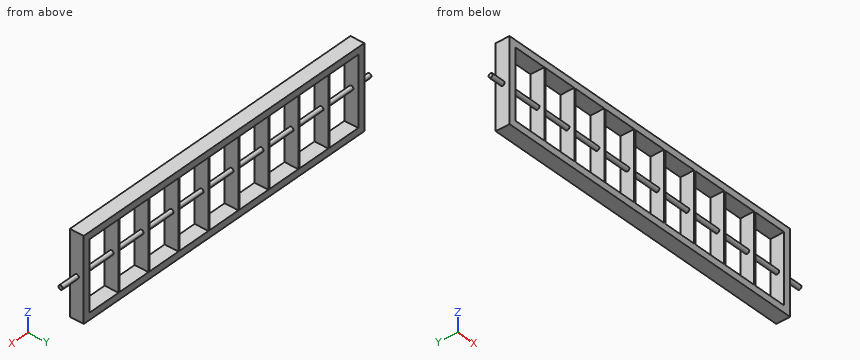
from build123d import *

# Parameters (mm, degrees)
SKETCH1_W                = 468
SKETCH1_H                = 120
SKETCH1_W_2              = 448
SKETCH1_H_2              = 100
BOSS_EXTRUDE1_DEPTH      = 20
SKETCH2_R                = 3
BOSS_EXTRUDE2_DEPTH      = 20
BOSS_EXTRUDE2_DEPTH_BACK = 495
SKETCH4_W                = 2
SKETCH4_H                = 20
BOSS_EXTRUDE3_DEPTH      = 100


with BuildPart() as part:
    # Sketch1 → Boss-Extrude1 (new body)
    with BuildSketch(Plane(origin=(0, 0, 0), x_dir=(1, 0, 0), z_dir=(0, 1, 0))):
        Rectangle(SKETCH1_W, SKETCH1_H)
        Rectangle(SKETCH1_W_2, SKETCH1_H_2, mode=Mode.SUBTRACT)
    extrude(amount=BOSS_EXTRUDE1_DEPTH)

    # Sketch2 → Boss-Extrude2 (add, two sides)
    with BuildSketch(Plane.ZY.offset(234)) as boss_extrude2_sk:
        with Locations((0, 10)):
            Circle(SKETCH2_R)
    extrude(amount=BOSS_EXTRUDE2_DEPTH)
    extrude(boss_extrude2_sk.sketch, amount=-BOSS_EXTRUDE2_DEPTH_BACK)

    # Sketch4 → Boss-Extrude3 (add)
    with BuildSketch(Plane(origin=(0, 0, 50), x_dir=(-1, 0, 0), z_dir=(0, 0, -1))):
        with Locations((-125, 10)):
            Rectangle(SKETCH4_W, SKETCH4_H)
        with Locations((-75, 10)):
            Rectangle(SKETCH4_W, SKETCH4_H)
        with Locations((-25, 10)):
            Rectangle(SKETCH4_W, SKETCH4_H)
        with Locations((25, 10)):
            Rectangle(SKETCH4_W, SKETCH4_H)
        with Locations((75, 10)):
            Rectangle(SKETCH4_W, SKETCH4_H)
        with Locations((125, 10)):
            Rectangle(SKETCH4_W, SKETCH4_H)
        with Locations((175, 10)):
            Rectangle(SKETCH4_W, SKETCH4_H)
        with Locations((-175, 10)):
            Rectangle(SKETCH4_W, SKETCH4_H)
    extrude(amount=BOSS_EXTRUDE3_DEPTH)


solid = part.part
Geometry check sheet. Reference: the model listing, model coordinates, mm. Coordinates: 2 decimals unless noted, no trailing zeros. Write each loop counter-clockwise with the first axis right and the second up, starting at its lowest first coordinate (ties: lowest second). Pieces come first, ordered by that corner, then holes. Notation, with made-up numbers: (-8.75, 74.25) -> (45.25, 74.25) arc R20 cw to (45.25, 82.25) -> close; hole circle Ø5 at (3, 12.5). An arc over 180 degrees is marked (long way). One line per question, with ' | ' between items.
1. Thickness scan on probe 1 along Z at (x, y) = (91, 3); probe 2 along Z at (x, y) = (-188, 12.5); probe 3 along X at (y, z) = (3.5, 52). Record the ranges inside material, lowest first. Write a range as from..to.
Answers:
probe 1: z = -60..-50, 50..60 | probe 2: z = -60..-50, -1.66..1.66, 50..60 | probe 3: x = -234..234
2. Depth check by flat-ended pin: pin 1 Ø8 at (y, z) = (2.5, -35.5) entering from -X; pin 2 Ø10 at (y, z) = (8.5, 17) entering from +X. Enter the tip coordinate at first touch or a pass-through.
Answers:
pin 1: stops at x = -234 | pin 2: stops at x = 234
3. Cross-section at B-B on y = 10. State how many separate pieces and enclosed holes the cut face has, and give its area (3 significant figures).
Answers:
separate pieces: 1 | enclosed holes: 18 | area: 15,800 mm²
4. Cross-section at A-A on x = 200. Record the cut outline in (y, z), and give its area (3 significant figures).
Answers:
outline: (0, -60) -> (20, -60) -> (20, -50) -> (0, -50) -> close; (0, 50) -> (20, 50) -> (20, 60) -> (0, 60) -> close; circle Ø6 at (10, 0) | area: 428 mm²
